Geometry check sheet. Reference: the model listing, model coordinates, mm. Face numbers are marked on the shaded views. A direction names the side the tool comes from. Coordinates: 2 decimals unless noted, no trailing zeros. Write each loop counter-clockwise with the first axis right and the second up, starting at its lowest first coordinate (ties: lowest second). Pieces come first, ordered by that corner, then holes. Notation, with made-up numbers: (65, -39) -> (110, -39) arc R8 cw to (110, -30) -> close; hole circle Ø1 at (22, -18). An arc over 180 degrees is marked (long way). Answer as CSV lines item,"result".
```python
from build123d import *

# Parameters (mm, degrees)
SKETCH1_W           = 44
SKETCH1_H           = 15
BOSS_EXTRUDE1_DEPTH = 5
SKETCH2_W           = 11.9
SKETCH2_H           = 15
BOSS_EXTRUDE2_DEPTH = 4
SKETCH3_R           = 1.55
CUT_EXTRUDE1_DEPTH  = 3
SKETCH4_R           = 1.55
CUT_EXTRUDE2_DEPTH  = 3
CUT_EXTRUDE3_DEPTH  = 3
SKETCH7_W           = 11.9
SKETCH7_H           = 6
CUT_EXTRUDE4_DEPTH  = 7
SKETCH8_W           = 11.9
SKETCH8_H           = 2.1
CUT_EXTRUDE5_DEPTH  = 3
SKETCH9_R           = 1.55
BOSS_EXTRUDE4_DEPTH = 1.5


with BuildPart() as part:
    # Sketch1 → Boss-Extrude1 (new body)
    with BuildSketch(Plane(origin=(0, 0, 0), x_dir=(1, 0, 0), z_dir=(0, 1, 0))):
        with Locations((22, -7.5)):
            Rectangle(SKETCH1_W, SKETCH1_H)
    extrude(amount=BOSS_EXTRUDE1_DEPTH)

    # Sketch2 → Boss-Extrude2 (add)
    with BuildSketch(Plane(origin=(0, 5, 0), x_dir=(1, 0, 0), z_dir=(0, 1, 0))):
        with Locations((22, -7.5)):
            Rectangle(SKETCH2_W, SKETCH2_H)
    extrude(amount=BOSS_EXTRUDE2_DEPTH)

    # Sketch3 → Cut-Extrude1 (cut)
    with BuildSketch(Plane(origin=(0, 5, 0), x_dir=(1, 0, 0), z_dir=(0, 1, 0))):
        with Locations((10, -10)):
            Circle(SKETCH3_R)
        with Locations((34, -10)):
            Circle(SKETCH3_R)
    extrude(amount=-CUT_EXTRUDE1_DEPTH, mode=Mode.SUBTRACT)

    # Sketch4 → Cut-Extrude2 (cut)
    with BuildSketch(Plane(origin=(0, 9, 0), x_dir=(1, 0, 0), z_dir=(0, 1, 0))):
        with Locations((22.05, -10)):
            Circle(SKETCH4_R)
    extrude(amount=-CUT_EXTRUDE2_DEPTH, mode=Mode.SUBTRACT)

    # Sketch6 → Cut-Extrude3 (cut)
    with BuildSketch(Plane(origin=(0, 5, 0), x_dir=(1, 0, 0), z_dir=(0, 1, 0))):
        Polygon((16.05, -4.8), (12.75, -4.8), (12.05, 0), (16.05, 0), align=None)
        Polygon((0, -15), (4.3, -15), (4.3, -11.4), (0, -9.8), align=None)
        Polygon((39.7, -11.4), (44, -9.8), (44, -15), (39.7, -15), align=None)
        Polygon((31.95, 0), (27.95, 0), (27.95, -4.8), (31.25, -4.8), align=None)
    extrude(amount=-CUT_EXTRUDE3_DEPTH, mode=Mode.SUBTRACT)

    # Sketch7 → Cut-Extrude4 (cut)
    with BuildSketch(Plane(origin=(0, 9, 0), x_dir=(1, 0, 0), z_dir=(0, 1, 0))):
        with Locations((22, -3)):
            Rectangle(SKETCH7_W, SKETCH7_H)
    extrude(amount=-CUT_EXTRUDE4_DEPTH, mode=Mode.SUBTRACT)

    # Sketch8 → Cut-Extrude5 (cut)
    with BuildSketch(Plane(origin=(0, 9, 0), x_dir=(1, 0, 0), z_dir=(0, 1, 0))):
        with Locations((22, -13.95)):
            Rectangle(SKETCH8_W, SKETCH8_H)
    extrude(amount=-CUT_EXTRUDE5_DEPTH, mode=Mode.SUBTRACT)

    # Sketch9 → Boss-Extrude4 (add)
    with BuildSketch(Plane(origin=(0, 5, 0), x_dir=(1, 0, 0), z_dir=(0, 1, 0))):
        Polygon((0, 0), (12.05, 0), (12.75, -4.8), (16.05, -4.8), (16.05, -15), (4.3, -15), (4.3, -11.4), (0, -9.8), align=None)
        with Locations((10, -10)):
            Circle(SKETCH9_R, mode=Mode.SUBTRACT)
        Polygon((39.7, -11.4), (44, -9.8), (44, 0), (31.95, 0), (31.25, -4.8), (27.95, -4.8), (27.95, -15), (39.7, -15), align=None)
        with Locations((34, -10)):
            Circle(SKETCH9_R, mode=Mode.SUBTRACT)
    extrude(amount=BOSS_EXTRUDE4_DEPTH)


solid = part.part
```
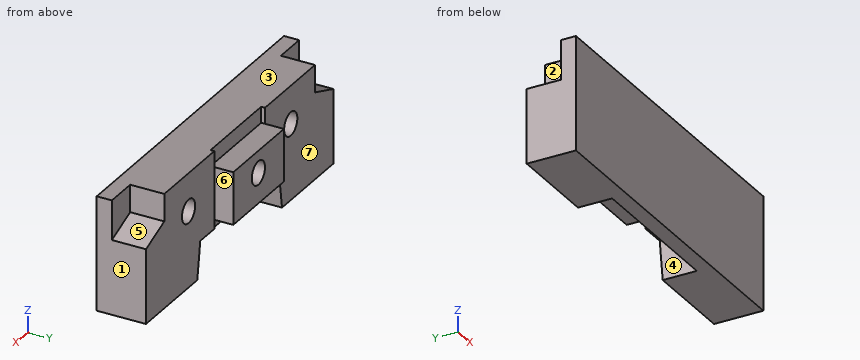
Item 1: Set-up check for the marked faces 5, 6 and 7: record each of +Z, -Z, +X, -X, +Y, -Y from which the full face is reachable in a straight line by a thin tool's end or side.
Responses:
face 5,"+Z, +X, +Y"
face 6,"+Z, -Z, +X, +Y"
face 7,"+Z, -Z, -X, +Y"
Item 2: Release check for a two-part mould opening along X. For the marked faces 1, 2, 3 and 4 record: +X half, -X half, draft (parallel to the pull), parting line (faces both ways), or undercut.
Responses:
face 1,"+X half"
face 2,"-X half"
face 3,"draft"
face 4,"undercut"
Item 3: Depth check by flat-ended pin: pin 1 Ø0.9 at (x, z) = (22.5, 9.5) entering from +Y; pin 2 Ø0.9 at (x, y) = (20.5, 7.5) entering from +Z; pin 3 Ø5 at (x, z) = (9.5, 2) entering from +Y. Enter the tip coordinate at first touch or a pass-through.
Responses:
pin 1,"stops at y = 6"
pin 2,"stops at z = 12.9"
pin 3,"stops at y = 6.5"
Item 4: Cross-section at C-C, the plane z = 5.5. Record the cut outline in (x, y), plus the area to 3 significant figures.
Responses:
outline,"(0, 0) -> (44, 0) -> (44, 6.5) -> (27.95, 6.5) -> (27.95, 2) -> (16.05, 2) -> (16.05, 6.5) -> (0, 6.5) -> close"
area,"232 mm2"
Item 5: Cross-section at B-B, the plane x = 22.05. Record the cut outline in (y, z).
Responses:
outline,"(0, 0) -> (2, 0) -> (2, 6) -> (9, 6) -> (9, 8.45) -> (6, 8.45) -> (6, 11.55) -> (9, 11.55) -> (9, 12.9) -> (6, 12.9) -> (6, 15) -> (0, 15) -> close"
Item 6: Thickness scan on probe 1 along Z at (x, y) = (34, 4.7); probe 2 along X at (y, z) = (8.25, 10); probe 3 along Y at (x, z) = (21, 4.75). Record the ranges inside material, lowest first.
Responses:
probe 1,"z = 0 to 8.45, 11.55 to 15"
probe 2,"x = 16.05 to 20.5, 23.6 to 27.95"
probe 3,"y = 0 to 2"
Item 7: Cross-section at D-D, the plane y = 7.25. Record the cut outline in (x, z).
Responses:
outline,"(16.05, 6) -> (27.95, 6) -> (27.95, 12.9) -> (16.05, 12.9) -> close; hole circle Ø3.1 at (22.05, 10)"
Item 8: Cross-section at A-A, the plane y = 3.25. Record the cut outline in (x, z), plus the area to 3 significant figures.
Responses:
outline,"(0, 0) -> (12.05, 0) -> (12.75, 4.8) -> (16.05, 4.8) -> (16.05, 6) -> (27.95, 6) -> (27.95, 4.8) -> (31.25, 4.8) -> (31.95, 0) -> (44, 0) -> (44, 9.8) -> (39.7, 11.4) -> (39.7, 15) -> (4.3, 15) -> (4.3, 11.4) -> (0, 9.8) -> close; hole circle Ø3.1 at (10, 10); hole circle Ø3.1 at (34, 10)"
area,"501 mm2"
